```python
from build123d import *

# Parameters (mm, degrees)
F0_W        = 3
F0_H        = 30
F1_DEPTH    = 30
F3_DEPTH    = 60
F4_T1_DEPTH = 60
F4_T3_DEPTH = 71.7271911209
F4_T5_DEPTH = 70
F4_T7_DEPTH = 67.3205080757


# Not quite as in the source:
# - a fillet or chamfer that OpenCascade refuses, or shapes differently, is made with other operations: its cross-section is extruded or revolved along the edge and cut away or added


with BuildPart() as f1:
    # F0 (on Front) → F1 (new body, symmetric)
    with BuildSketch(Plane.XZ):
        Polygon((13, -25), (16, -25), (16, 10), (13, 10), (-13, 10), (-16, 10), (-16, -25), (-9, -25), (-13, 0), (13, 0), align=None)
        with Locations((-14.5, 25)):
            Rectangle(F0_W, F0_H)
        with Locations((14.5, 25)):
            Rectangle(F0_W, F0_H)
    extrude(amount=F1_DEPTH, both=True)

    # F2 (on face) → F3 (cut, through all)
    with BuildSketch(Plane.XZ.offset(30)):
        with BuildLine():
            Line((9, 0), (13, 0))
            ThreePointArc((13, 0), (11, 2), (9, 0))
        make_face()
    extrude(amount=-F3_DEPTH, mode=Mode.SUBTRACT)

    # F4: fillet of radius 2 on 13 edges, made by hand

    # F4_s2 → F4_t1 (join)
    with BuildSketch(Plane.XZ.offset(-30)):
        with BuildLine():
            ThreePointArc((-10.6545617758, 0), (-12.1763965245, -0.7023024244), (-12.6294430396, -2.3159810022))
            Line((-12.6294430396, -2.3159810022), (-13, 0))
            Line((-13, 0), (-10.6545617758, 0))
        make_face()
        with BuildLine():
            ThreePointArc((-13, 12), (-12.4142135624, 10.5857864376), (-11, 10))
            Line((-11, 10), (-13, 10))
            Line((-13, 10), (-13, 12))
        make_face()
        with BuildLine():
            ThreePointArc((11, 10), (12.4142135624, 10.5857864376), (13, 12))
            Line((13, 12), (13, 10))
            Line((13, 10), (11, 10))
        make_face()
    extrude(amount=F4_T1_DEPTH)

    # F4_s4 → F4_t3 (cut)
    with BuildSketch(Plane.XZ.offset(-35.8635955605)):
        with BuildLine():
            ThreePointArc((-9.3705569604, -22.6840189978), (-9.8236034755, -24.2976975756), (-11.3454382242, -25))
            Line((-11.3454382242, -25), (-9, -25))
            Line((-9, -25), (-9.3705569604, -22.6840189978))
        make_face()
    extrude(amount=F4_T3_DEPTH, mode=Mode.SUBTRACT)

    # F4_s6 → F4_t5 (cut)
    with BuildSketch(Plane.XZ.offset(-35)):
        with BuildLine():
            ThreePointArc((-14, -25), (-15.4142135624, -24.4142135624), (-16, -23))
            Line((-16, -23), (-16, -25))
            Line((-16, -25), (-14, -25))
        make_face()
        with BuildLine():
            ThreePointArc((14, -25), (15.4142135624, -24.4142135624), (16, -23))
            Line((16, -23), (16, -25))
            Line((16, -25), (14, -25))
        make_face()
        with BuildLine():
            ThreePointArc((-15, 40), (-13.5857864376, 39.4142135624), (-13, 38))
            Line((-13, 38), (-13, 40))
            Line((-13, 40), (-15, 40))
        make_face()
        with BuildLine():
            ThreePointArc((-16, 38), (-15.4142135624, 39.4142135624), (-14, 40))
            Line((-14, 40), (-16, 40))
            Line((-16, 40), (-16, 38))
        make_face()
        with BuildLine():
            ThreePointArc((16, 38), (15.4142135624, 39.4142135624), (14, 40))
            Line((14, 40), (16, 40))
            Line((16, 40), (16, 38))
        make_face()
        with BuildLine():
            ThreePointArc((13, 38), (13.5857864376, 39.4142135624), (15, 40))
            Line((15, 40), (13, 40))
            Line((13, 40), (13, 38))
        make_face()
        with BuildLine():
            ThreePointArc((15, -25), (13.5857864376, -24.4142135624), (13, -23))
            Line((13, -23), (13, -25))
            Line((13, -25), (15, -25))
        make_face()
    extrude(amount=F4_T5_DEPTH, mode=Mode.SUBTRACT)

    # F4_s8 → F4_t7 (cut)
    with BuildSketch(Plane.XZ.offset(-33.6602540378)):
        with BuildLine():
            ThreePointArc((9.2679491924, 1), (8.5358983849, 0.2679491924), (7.5358983849, 0))
            Line((7.5358983849, 0), (9, 0))
            ThreePointArc((9, 0), (9.0681483474, 0.5176380902), (9.2679491924, 1))
        make_face()
    extrude(amount=F4_T7_DEPTH, mode=Mode.SUBTRACT)


solid = f1.part
```
Here's how the part is built. I have some questions about the finished solid (model axes, mm). A direction names the side the tool comes from. Give positions to 0.01 mm unless a question says otherwise; leave off trailing zeros. Order: outer loops, then holes, each group sorted by start corner. A loop starts at its lowest first (then second) coordinate and runs counter-clockwise, first axis right, second up. Notation, with made-up numbers: M -35,-24 L -7,-24 A6 ccw -7,-19 Z; hole C 34,55 d2. An arc over 180 degrees is marked long. Use a Markdown table: item, result. Add a question column.
1. On a 3-axis mill with a long thin cutter (end or side, diameter ignored), from which of +Z, -Z, +X, -X, +Y, -Y can I reach the whole of each face in a straight line? I mean faces 1 (the flat face through (-16, 0, 8)), 2 (the cylindrical face through (15.6, 0.4, -24.2)), 3 (the flat face through (0, 0, 10)), 4 (the cylindrical face through (-12.161, 0.42, -0.684)), 5 (the cylindrical face through (13.4, 0.4, -24.2)). Say none if no direction works.
2. Suppose I cut it at A-A (z = -5). List the corners of the cut face in (x, y) for me.
3. Suppose I cut it at D-D (x = -1). List the corners of the cut face in (y, z) for me.
4. For pin 1 Ø6 at (x, y) = (-4.5, -6.5) entering from -Z; pin 2 Ø6 at (x, y) = (-8, 10) entering from -Z; pin 3 Ø11 at (x, y) = (-4, -7) entering from +Z; pin 4 Ø10 at (x, z) = (-4, -18) entering from +Y, each with a flat end and sliding along its axis, tell me the tip position at first contact or that it passes through.
5. Suppose I cut it at B-B (y = 15.5). List the corners of the cut face in (x, z) for me.
6. I need wall thicknesses on probe 1 along X at (y, z) = (-3.5, 37.5); probe 2 along Z at (x, y) = (-2.5, -8); probe 3 along X at (y, z) = (6.5, -16). Which ranges of each line are inside material? Lowest first, please. Write a range as from..to.
7. Suppose I cut it at C-C (z = 18). List the corners of the cut face in (x, y) for me.
8. If we mould it in two halves opening along X, with no side actions, what happens to faces 6 (the flat face through (0, -30, 8)), 7 (the cylindrical face through (15.6, 0.4, 39.2)), 8 (the cylindrical face through (-13.4, 0.4, 39.2)), 9 (the cylindrical face through (-15.4, 0.42, -24.43))? For each: +X half, -X half, draft (parallel to the pull), parting line (faces both ways), or undercut.
Results list:
| question | item | result |
|---|---|---|
| 1 | face 1 | +Z, -Z, -X, +Y, -Y |
| 1 | face 2 | -Z, +X, +Y, -Y |
| 1 | face 3 | +Z, +Y, -Y |
| 1 | face 4 | +Y, -Y |
| 1 | face 5 | -Z, +Y, -Y |
| 2 | outline | M -16,-30 L -12.2,-30 L -12.2,30 L -16,30 Z; M 13,-30 L 16,-30 L 16,30 L 13,30 Z |
| 3 | outline | M -30,0 L 30,0 L 30,10 L -30,10 Z |
| 4 | pin 1 | stops at z = 0 |
| 4 | pin 2 | stops at z = -24.97 |
| 4 | pin 3 | stops at z = 10 |
| 4 | pin 4 | passes through |
| 5 | outline | M -16,-23 A2 ccw -14,-25 L -11.35,-25 A2 ccw -9.37,-22.68 L -12.63,-2.32 A2 cw -10.65,0 L 7.54,0 A2 ccw 9.27,1 A2 cw 13,0 L 13,-23 A2 ccw 14.5,-24.94 A2 ccw 16,-23 L 16,38 A2 ccw 14.5,39.94 A2 ccw 13,38 L 13,12 A2 cw 11,10 L -11,10 A2 cw -13,12 L -13,38 A2 ccw -14.5,39.94 A2 ccw -16,38 Z |
| 6 | probe 1 | x = -16..-13, 13..16 |
| 6 | probe 2 | z = 0..10 |
| 6 | probe 3 | x = -16..-10.44, 13..16 |
| 7 | outline | M -16,-30 L -13,-30 L -13,30 L -16,30 Z; M 13,-30 L 16,-30 L 16,30 L 13,30 Z |
| 8 | face 6 | draft |
| 8 | face 7 | +X half |
| 8 | face 8 | undercut |
| 8 | face 9 | -X half |
